from build123d import *

# Parameters (mm, degrees)
F2_DEPTH = 5
F3_DEPTH = 30


with BuildPart() as f2:
    # F0 (on Top) → F2 (new body)
    with BuildSketch(Plane.XY):
        with BuildLine():
            ThreePointArc((-10, 0), (0, 10), (10, 0))
            Line((10, 0), (37, 0))
            ThreePointArc((37, 0), (47, 10), (57, 0))
            Line((57, 0), (62, 0))
            Line((62, 0), (62, 15))
            Line((62, 15), (-15, 15))
            Line((-15, 15), (-15, 0))
            Line((-15, 0), (-10, 0))
        make_face()
        with BuildLine():
            Line((37, 0), (10, 0))
            ThreePointArc((10, 0), (0, -10), (-10, 0))
            Line((-10, 0), (-15, 0))
            Line((-15, 0), (-15, -15))
            Line((-15, -15), (62, -15))
            Line((62, -15), (62, 0))
            Line((62, 0), (57, 0))
            ThreePointArc((57, 0), (47, -10), (37, 0))
        make_face()
    extrude(amount=F2_DEPTH)

    # F0 (on Top) → F3 (join)
    with BuildSketch(Plane.XY):
        with BuildLine():
            ThreePointArc((-10, 0), (0, -10), (10, 0))
            Line((10, 0), (0, 0))
            Line((0, 0), (-10, 0))
        make_face()
        with BuildLine():
            Line((0, 0), (10, 0))
            ThreePointArc((10, 0), (0, 10), (-10, 0))
            Line((-10, 0), (0, 0))
        make_face()
        with BuildLine():
            Line((47, 0), (37, 0))
            ThreePointArc((37, 0), (47, -10), (57, 0))
            Line((57, 0), (47, 0))
        make_face()
        with BuildLine():
            ThreePointArc((57, 0), (47, 10), (37, 0))
            Line((37, 0), (47, 0))
            Line((47, 0), (57, 0))
        make_face()
    extrude(amount=F3_DEPTH)


solid = f2.part
The model under review builds one solid part; all positions refer to its coordinate system, in mm. A direction names the side the tool comes from. Coordinates: 2 decimals unless noted, no trailing zeros. Loops run counter-clockwise (first coordinate to the right, second up) from the corner with the lowest first, then second, coordinate; pieces in that order, holes last. Notation, with made-up numbers: M 53,1 L 90,1 A36 ccw 90,38 Z; hole C 35,-17 d10. An arc over 180 degrees is marked long. Put each result on its own line as item: value. Start each with the question number.
Q1. Add section A-A (x = 47). Write out the cut boundary in (y, z).
Q2. Clearance check with flat-ended pins moving along their axes: pin 1 (1.5 mm diameter, centred on x = 48, y = 11.5, fed in from -Z); pin 2 (4 mm diameter, centred on x = 33.5, y = 9.5, fed in from +Z); pin 3 (5 mm diameter, centred on y = -2, z = 24, fed in from -X); pin 4 (2 mm diameter, centred on y = -8, z = 22.5, fed in from +X). State where each tip first meets the part, or that it passes through.
Q3. Add section B-B (z = 20.5). Write out the cut boundary in (x, y), and give its area (3 significant figures).
Q4. For faces 1 (the flat face through (62, 0, 2)), 2 (the cylindrical face through (-8, -6, 17)), list the 3-axis set-ups (+Z, -Z, +X, -X, +Y, -Y) from which the entire face can be reached by the end or side of a thin tool; tool diameter is ignored.
Q5. The part is to be moulded in two halves that separate along X. For faces 3 (the flat face through (23, 0, 5)), 4 (the flat face through (-15, 0, 2)), 5 (the flat face through (47, 0, 30)), say which applies: +X half, -X half, draft (parallel to the pull), parting line (faces both ways), or undercut.
Q6. Wall thickness on line 1 (Z direction, x = 11.5, y = -9.5); line 2 (X direction, y = -5.75, z = 23); line 3 (X direction, y = 7.75, z = 22.25): over which ranges is each line inside the solid? List them lowest first.
Q7. Add section C-C (y = 0). Write out the cut boundary in (x, z).
Q8. Add section D-D (x = 5.5). Write out the cut boundary in (y, z), and give its area (3 significant figures).
Answers:
1. outline: M -15,0 L 15,0 L 15,5 L 10,5 L 10,30 L -10,30 L -10,5 L -15,5 Z
2. pin 1: stops at z = 0
2. pin 2: stops at z = 5
2. pin 3: stops at x = -10
2. pin 4: stops at x = 54.14
3. outline: C 0,0 d20; C 47,0 d20
3. area: 628 mm^2
4. face 1: +Z, -Z, +X, +Y, -Y
4. face 2: +Z
5. face 3: undercut
5. face 4: -X half
5. face 5: draft
6. line 1: z = 0 to 5
6. line 2: x = -8.18 to 8.18, 38.82 to 55.18
6. line 3: x = -6.32 to 6.32, 40.68 to 53.32
7. outline: M -15,0 L 62,0 L 62,5 L 57,5 L 57,30 L 37,30 L 37,5 L 10,5 L 10,30 L -10,30 L -10,5 L -15,5 Z
8. outline: M -15,0 L 15,0 L 15,5 L 8.35,5 L 8.35,30 L -8.35,30 L -8.35,5 L -15,5 Z
8. area: 568 mm^2
